Input: dimensioned drawing with shaded views. Units: mm. Origin: part minimum x, y, z. A direction names the side the tool comes from. Give positions to 0.01 mm unless a question says otherwise; leave off trailing zeros. Order: outer loops, then holes, each group sorted by start corner. A loop starts at its lowest first (then second) coordinate and runs counter-clockwise, first axis right, second up. Notation, with made-up numbers: (-24, 34) -> (24, 34) arc R4 cw to (24, 41) -> close; hole circle Ø1 at (-24, 86). An arc over 180 degrees is marked (long way). One line per question, with ' | ' between items. Start each with the question number.
(1) Ray query, L1, parallel to Y at x = 14, z = 1.75 (1 decimal); L2, parallel to Z at x = 21.75, y = 28.5; L3, parallel to Y at x = 14.5, z = 4 (1 decimal). Return the intervals inside material, ascending.
(2) Set-up query: the marked faces 1 and 2. Return all of +Z, -Z, +X, -X, +Y, -Y with unobstructed straight access to the full face (end or side cutting, diameter ignored); none if empty.
(3) First-contact query: pin 1 Ø5 at (x, y) = (14, 13.7) entering from -Z; pin 2 Ø2 at (x, z) = (15, 3) entering from -Y. Flat tips, straight axial feed; report the tip coordinate or a pass-through.
(4) Section D-D (x = 6.25). Return loops of the section in (y, z).
(5) Section A-A (x = 14). State how many separate pieces and enclosed holes the cut face has.
(6) Section B-B (y = 64.5). Return loops of the section in (x, z) (1 decimal).
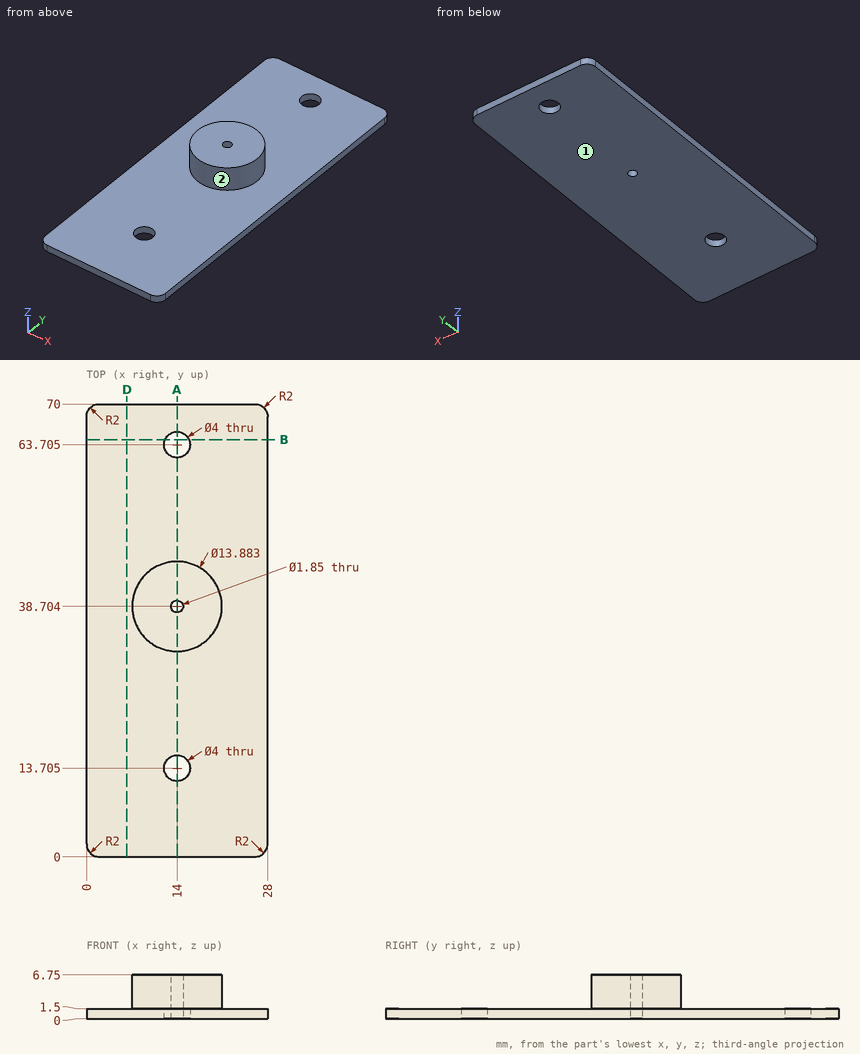
Response:
1) L1: y = 31.8 to 37.8, 39.6 to 45.6 | L2: z = 0 to 1.5 | L3: y = 31.8 to 37.9, 39.5 to 45.6
2) face 1: -Z, +X, -X, +Y, -Y | face 2: +Z
3) pin 1: stops at z = 0 | pin 2: stops at y = 31.76
4) outline: (0, 0) -> (70, 0) -> (70, 1.5) -> (0, 1.5) -> close
5) separate pieces: 4 | enclosed holes: 0
6) outline: (0, 0) -> (12.2, 0) -> (12.2, 1.5) -> (0, 1.5) -> close; (15.8, 0) -> (28, 0) -> (28, 1.5) -> (15.8, 1.5) -> close
